Verification items for the finished model (mm, model axes). Face numbers are marked on the shaded views. A direction names the side the tool comes from. Round coordinates to 2 decimals unless told otherwise and drop trailing zeros. Write each loop counter-clockwise with the first axis right and the second up, starting at its lowest first coordinate (ties: lowest second). Pieces come first, ordered by that corner, then holes. Notation, with made-up numbers: (59.25, 78) - (64.25, 78) arc R14 ccw to (64.25, 91) - close; hole circle Ø7 at (-18, 60.25). An arc over 180 degrees is marked (long way). Answer as a JSON object with one key per item and string values. Group by question number.
1) Set-up check for the marked faces 1, 2 and 3: record each of +Z, -Z, +X, -X, +Y, -Y from which the full face is reachable in a straight line by a thin tool's end or side.
2) Section check A-A (y = 13). Enter the section's corners in (x, z) (3 decimals), then the cut area to 3 significant figures.
3) Section check C-C (z = -30.5). Enter the section's corners in (x, y) (1 decimal).
4) Go/stop test with flat-tipped pins: pin 1 Ø5 at (x, y) = (4, 28.5) entering from -Z; pin 2 Ø0.5 at (y, z) = (21, 6) entering from -X; pin 3 Ø2 at (x, z) = (7.5, -29.5) entering from +Y. Record where each tip stops, or that it passes through.
5) Thickness scan on line 1 (Z direction, x = 7, y = 2); line 2 (Y direction, x = 4.5, z = -14); line 3 (Y direction, x = 3.5, z = -5). Record the ranges inside material, lowest first.
6) Mould release check, pull along Y, two halves, no side actions. Record for the marked faces 4, 5 and 6: +Y half, -Y half, draft (parallel to the pull), parting line (faces both ways), or undercut.
7) Section check B-B (z = -5). Enter the section's corners in (x, y) (3 decimals).
```python
from build123d import *

# Parameters (mm, degrees)
BASE_SKETCH_W           = 13.3096
BASE_SKETCH_H           = 27.94
BASE_DEPTH              = 19.6977
MOUNTING_POINT_SKETCH_W = 13.3096
MOUNTING_POINT_SKETCH_H = 40.386
MOUNTING_POINT_DEPTH    = 1.7526
MOUNTING_HOLES_DEPTH    = 22.4503
MIDDLE_SKETCH_W         = 13.3096
MIDDLE_SKETCH_H         = 27.94
MIDDLE_DEPTH            = 4.9911
TOP_EXTRUDE_DEPTH       = 3.1496
GEAR_SKETCH_R           = 2.9083
GEAR_DEPTH              = 4.2418
SERVO_CABLE_SKETCH_W    = 5.3594
SERVO_CABLE_SKETCH_H    = 3.6576
SEVO_CABLE_DEPTH        = 5.1562
FILLET1_R               = 0.635


with BuildPart() as part:
    # Base Sketch → Base (new body)
    with BuildSketch(Plane(origin=(0, 0, 0), x_dir=(1, 0, 0), z_dir=(0, 1, 0))):
        with Locations((6.6548, 13.97)):
            Rectangle(BASE_SKETCH_W, BASE_SKETCH_H)
    extrude(amount=BASE_DEPTH)

    # Mounting Point Sketch → Mounting Point (add)
    with BuildSketch(Plane(origin=(0, 19.6977, 0), x_dir=(1, 0, 0), z_dir=(0, 1, 0))):
        with Locations((6.6548, 13.97)):
            Rectangle(MOUNTING_POINT_SKETCH_W, MOUNTING_POINT_SKETCH_H)
    extrude(amount=MOUNTING_POINT_DEPTH)

    # Mounting Holes Sketch → Mounting Holes (cut, through all)
    with BuildSketch(Plane(origin=(0, 21.4503, 0), x_dir=(1, 0, 0), z_dir=(0, 1, 0))):
        with BuildLine():
            Line((5.6769, 34.163), (7.6327, 34.163))
            Line((7.6327, 34.163), (7.6327, 32.37744567))
            ThreePointArc((7.6327, 32.37744567), (6.6548, 29.0449), (5.6769, 32.37744567))
            Line((5.6769, 32.37744567), (5.6769, 34.163))
        make_face()
        with BuildLine():
            Line((5.6769, -6.223), (7.6327, -6.223))
            Line((7.6327, -6.223), (7.6327, -4.43744567))
            ThreePointArc((7.6327, -4.43744567), (6.6548, -1.1049), (5.6769, -4.43744567))
            Line((5.6769, -4.43744567), (5.6769, -6.223))
        make_face()
    extrude(amount=-MOUNTING_HOLES_DEPTH, mode=Mode.SUBTRACT)

    # Middle Sketch → Middle (add)
    with BuildSketch(Plane(origin=(0, 21.4503, 0), x_dir=(1, 0, 0), z_dir=(0, 1, 0))):
        with Locations((6.6548, 13.97)):
            Rectangle(MIDDLE_SKETCH_W, MIDDLE_SKETCH_H)
    extrude(amount=MIDDLE_DEPTH)

    # Top Sketch → Top extrude (add)
    with BuildSketch(Plane(origin=(0, 26.4414, 0), x_dir=(1, 0, 0), z_dir=(0, 1, 0))):
        with BuildLine():
            Line((0, 27.94), (13.3096, 27.94))
            Line((13.3096, 27.94), (13.3096, 13.6525))
            Line((13.3096, 13.6525), (10.4775, 13.6525))
            ThreePointArc((10.4775, 13.6525), (6.6548, 9.8298), (2.8321, 13.6525))
            Line((2.8321, 13.6525), (0, 13.6525))
            Line((0, 13.6525), (0, 27.94))
        make_face()
    extrude(amount=TOP_EXTRUDE_DEPTH)

    # Gear Sketch → Gear (add)
    with BuildSketch(Plane(origin=(0, 29.591, 0), x_dir=(1, 0, 0), z_dir=(0, 1, 0))):
        with Locations((6.6548, 20.79625)):
            Circle(GEAR_SKETCH_R)
    extrude(amount=GEAR_DEPTH)

    # Servo Cable Sketch → Sevo Cable (add)
    with BuildSketch(Plane(origin=(0, 0, -27.94), x_dir=(-1, 0, 0), z_dir=(0, 0, -1))):
        with Locations((-6.6548, 5.5626)):
            Rectangle(SERVO_CABLE_SKETCH_W, SERVO_CABLE_SKETCH_H)
    extrude(amount=SEVO_CABLE_DEPTH)

    # Fillet1
    fillet1_edges = [part.edges().sort_by_distance(p)[0] for p in [
        (13.3096, 19.6977, 3.1115),
        (0, 9.84885, -27.94),
        (0, 19.6977, -31.0515),
        (0, 20.574, -34.163),
        (0, 21.4503, -31.0515),
        (0, 25.52065, -27.94),
        (0, 29.591, -20.79625),
        (0, 28.0162, -13.6525),
        (0, 26.4414, -6.82625),
        (0, 23.94585, 0),
        (0, 21.4503, 3.1115),
        (0, 20.574, 6.223),
        (0, 19.6977, 3.1115),
        (0, 0, -13.97),
        (0, 9.84885, 0),
        (6.6548, 19.6977, 0),
        (13.3096, 9.84885, 0),
        (6.6548, 0, 0),
        (9.3345, 5.5626, -33.0962),
        (6.6548, 3.7338, -33.0962),
        (3.9751, 5.5626, -33.0962),
        (6.6548, 7.3914, -33.0962),
        (3.9751, 7.3914, -30.5181),
        (3.9751, 3.7338, -30.5181),
        (9.3345, 3.7338, -30.5181),
        (9.3345, 7.3914, -30.5181),
        (6.6548, 0, -27.94),
        (13.3096, 9.84885, -27.94),
        (13.3096, 29.591, -20.79625),
        (13.3096, 23.94585, 0),
        (6.6548, 26.4414, 0),
        (13.3096, 26.4414, -6.82625),
        (11.89355, 29.591, -13.6525),
        (1.41605, 29.591, -13.6525),
        (6.6548, 29.591, -9.8298),
        (6.6548, 29.591, -27.94),
        (13.3096, 25.52065, -27.94),
        (13.3096, 20.574, -34.163),
    ]]
    fillet(fillet1_edges, radius=FILLET1_R)


solid = part.part
```
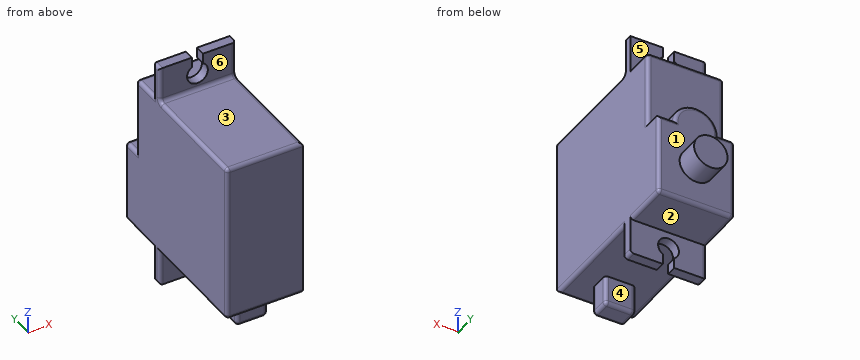
Returned:
{
 "1": {"face 1": "+Y", "face 2": "-Z, +X, -X, +Y", "face 3": "+Z, +X, -X, -Y"},
 "2": {"outline": "(0, -27.305) arc R0.635 ccw to (0.635, -27.94) - (12.675, -27.94) arc R0.635 ccw to (13.31, -27.305) - (13.31, -0.635) arc R0.635 ccw to (12.675, 0) - (0.635, 0) arc R0.635 ccw to (0, -0.635) - close", "area": "372 mm2"},
 "3": {"outline": "(0, 20.3) arc R0.6 ccw to (0.6, 19.7) - (4.9, 19.7) - (4.9, 21.5) - (0.6, 21.5) arc R0.6 ccw to (0, 20.8) - close; (4, 4.4) arc R0.6 ccw to (4.6, 3.7) - (8.7, 3.7) arc R0.6 ccw to (9.3, 4.4) - (9.3, 6.8) arc R0.6 ccw to (8.7, 7.4) - (4.6, 7.4) arc R0.6 ccw to (4, 6.8) - close; (8.4, 19.7) - (13.3, 19.7) - (13.3, 21.5) - (8.4, 21.5) - close"},
 "4": {"pin 1": "z = -27.94", "pin 2": "x = 0.02", "pin 3": "y = 21.45"},
 "5": {"line 1": "-27.94 to 0", "line 2": "0 to 29.59", "line 3": "0 to 26.44"},
 "6": {"face 4": "undercut", "face 5": "+Y half", "face 6": "-Y half"},
 "7": {"outline": "(0, 0.635) arc R0.635 ccw to (0.635, 0) - (13.31, 0) - (13.31, 25.806) arc R0.635 ccw to (12.675, 26.441) - (0.635, 26.441) arc R0.635 ccw to (0, 25.806) - close"}
}
